Check sheet for the modelled part. Datum: model origin and axes. Units: mm. Face numbers are marked on the shaded views. A direction names the side the tool comes from. Round coordinates to 2 decimals unless told otherwise and drop trailing zeros. Loops run counter-clockwise (first coordinate to the right, second up) from the corner with the lowest first, then second, coordinate; pieces in that order, holes last. Notation, with made-up numbers: (67, -35.5) -> (118, -35.5) arc R9 cw to (118, -31.5) -> close; hole circle Ø3 at (-36.75, -29.5). An arc over 180 degrees is marked (long way). One line per item, written item: value. Start each with the question number.
1. Material ranges on L1, parallel to Z at x = 27.5, y = 90; L2, parallel to X at y = 53.5, z = 16; L3, parallel to Y at x = -11, z = 15.5, recorded low to high.
2. Go/stop test with flat-tipped pins: pin 1 (3.5 mm diameter, centred on y = 63, z = 16, fed in from -X); pin 2 (3 mm diameter, centred on x = 70, z = 3, fed in from +Y); pin 3 (1 mm diameter, centred on y = -2.5, z = -15, fed in from +X); pin 4 (8 mm diameter, centred on x = 58, z = -8, fed in from -Y). Record where each tip stops, or that it passes through.
3. Set-up check for the marked faces 1 and 2: record each of +Z, -Z, +X, -X, +Y, -Y from which the full face is reachable in a straight line by a thin tool's end or side.
4. Cross-section at A-A on x = 76. Record the cut outline in (y, z).
5. Cross-section at C-C on x = -4.5. Record the cut outline in (y, z).
6. Cross-section at B-B on y = 48.5. Record the cut outline in (x, z), then the cut area to 3 significant figures.
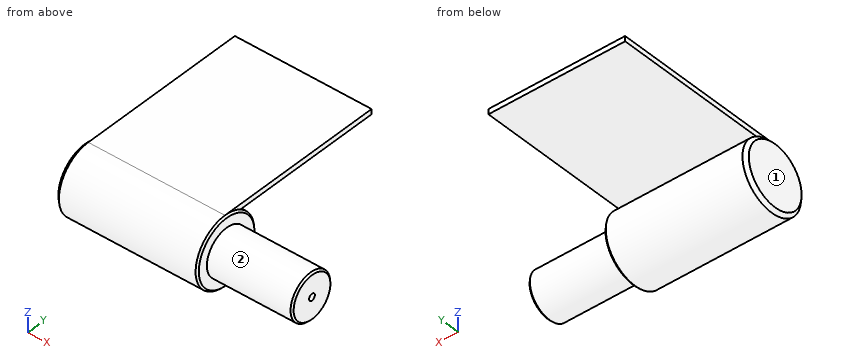
from build123d import *

# Parameters (mm, degrees)
SKETCH_3_W      = 80
SKETCH_3_H      = 3.000052495
EXTRUDE_1_DEPTH = 100


with BuildPart() as part:
    # Эскиз2 → Повернуть1 (revolve)
    with BuildSketch(Plane(origin=(0, 0, 0), x_dir=(1, 0, 0), z_dir=(0, 1, 0)), mode=Mode.PRIVATE) as revolve_1_sk:
        Polygon((-45.527497303, 22.337527379), (34.472502697, 22.337527379), (35.472502697, 21.337527379), (35.472502697, 15.837527379), (84.472502697, 15.837527379), (85.441558376, 14.8684717), (85.441558376, 4.296423316), (82.259183132, 2.337527379), (-47.527497303, 2.337527379), (-47.527497303, 20.337527379), align=None)
    revolve(revolve_1_sk.sketch.rotate(Axis((-58.608041749, 0, -2.337527379), (1, 0, 0)), 180), axis=Axis((-58.608041749, 0, -2.337527379), (1, 0, 0)))

    # Эскиз3 → Бобышка-Вытянуть1 (add)
    with BuildSketch(Plane(origin=(0, 0, 0), x_dir=(1, 0, 0), z_dir=(0, 1, 0))):
        with Locations((-5.527497303, -16.162446374)):
            Rectangle(SKETCH_3_W, SKETCH_3_H)
    extrude(amount=EXTRUDE_1_DEPTH)


solid = part.part
Taken from the geometry:
1. L1: z = 14.66 to 17.66
1. L2: x = -45.53 to 34.47
1. L3: y = -9.05 to 100
2. pin 1: stops at x = -45.53
2. pin 2: stops at y = 12.94
2. pin 3: stops at x = 85.44
2. pin 4: stops at y = -13.4
3. face 1: +Z, -Z, -X, +Y, -Y
3. face 2: +X
4. outline: circle Ø27 at (0, -2.34)
5. outline: (0, 17.66) arc R20 ccw (long way) to (10.54, 14.66) -> (100, 14.66) -> (100, 17.66) -> close
6. outline: (-45.53, 14.66) -> (34.47, 14.66) -> (34.47, 17.66) -> (-45.53, 17.66) -> close
6. area: 240 mm2
